The model under review builds one solid part; all positions refer to its coordinate system, in mm. Coordinates: 2 decimals unless noted, no trailing zeros. Loops run counter-clockwise (first coordinate to the right, second up) from the corner with the lowest first, then second, coordinate; pieces in that order, holes last. Notation, with made-up numbers: (64, 36) - (68, 36) arc R26 cw to (68, 67) - close; hole circle Ø9 at (-19.75, 14). An arc over 180 degrees is marked (long way). Answer in a Markdown table with one row per item. Add a question column.
(1) For P1, Ø8, axis at x = 0, y = 118.5, coming from the +Z side; P2, Ø6, axis at x = -118.5, y = 0, coming from the -Z side; P3, Ø1.5, axis at y = -96, z = 4.5, coming from the +X side; P4, Ø1.5, axis at x = -12, z = 1.5, coming from the -Y side, all flat-tipped, find the tip position at first contact; note any pin that passes through.
(2) We need section B-B on x = 25. Write out the cut boundary in (y, z), plus the area to 3 significant figures.
(3) We need section A-A on y = 92.5. Write out the cut boundary in (x, z), plus the area to 3 significant figures.
(4) For line 1 along Y through (x, z) = (0, 2.6); line 2 along Y through (x, z) = (0, 6.25); line 3 along Y through (x, z) = (-32, 6), list the stretches that pass through material, from the lowest coordinate up.
(5) We need section C-C on z = 4.25. Write out the cut boundary in (x, y), plus the area to 3 significant figures.
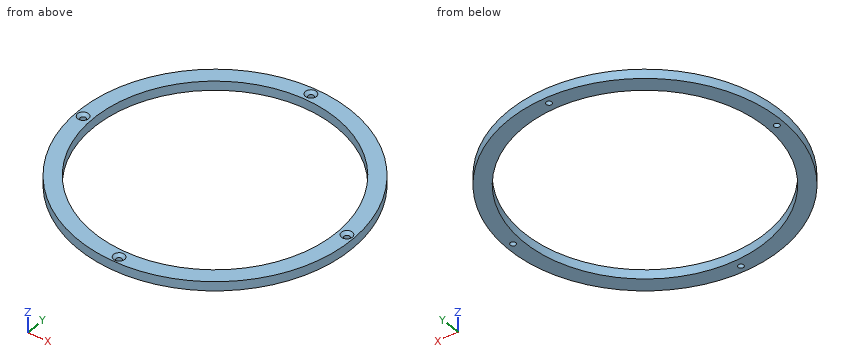
from build123d import *

# Parameters (mm, degrees)
SCHIZZO1_R                                           = 125
SCHIZZO1_R_2                                         = 111
ESTRUSIONE_ESTRUSIONE1_DEPTH                         = 8.5
FORO_SVASATO_PER_VITE_M4_A_TESTA_SVASATA_D           = 5
FORO_SVASATO_PER_VITE_M4_A_TESTA_SVASATA_CSINK_D     = 10
FORO_SVASATO_PER_VITE_M4_A_TESTA_SVASATA_CSINK_ANGLE = 90
RIPETIZIONECIRCOLARE1_COUNT                          = 4


with BuildPart() as part:
    # Schizzo1 → Estrusione-Estrusione1 (new body)
    with BuildSketch(Plane.XY):
        Circle(SCHIZZO1_R)
        Circle(SCHIZZO1_R_2, mode=Mode.SUBTRACT)
    extrude(amount=ESTRUSIONE_ESTRUSIONE1_DEPTH)

    # Foro svasato per Vite M4 a testa svasata cilindrica2 (through all)
    with Locations(Plane.XY.offset(8.5)):
        with Locations((0, -118.5)):
            foro_svasato_per_vite_m4_a_testa_svasata = CounterSinkHole(FORO_SVASATO_PER_VITE_M4_A_TESTA_SVASATA_D / 2, FORO_SVASATO_PER_VITE_M4_A_TESTA_SVASATA_CSINK_D / 2, counter_sink_angle=FORO_SVASATO_PER_VITE_M4_A_TESTA_SVASATA_CSINK_ANGLE)

    # RipetizioneCircolare1: Foro svasato per Vite M4 a testa svasata cilindrica2 ×4 about axis
    ripetizionecircolare1_axis = Axis((0, 0, 0), (0, 0, 1))
    for i in range(1, RIPETIZIONECIRCOLARE1_COUNT):
        add(foro_svasato_per_vite_m4_a_testa_svasata.rotate(ripetizionecircolare1_axis, i * 360 / RIPETIZIONECIRCOLARE1_COUNT), mode=Mode.SUBTRACT)


solid = part.part
Outcome:
| question | item | result |
|---|---|---|
| 1 | P1 | z = 7.5 |
| 1 | P2 | z = 0 |
| 1 | P3 | x = 80.95 |
| 1 | P4 | y = -124.49 |
| 2 | outline | (-122.47, 0) - (-108.15, 0) - (-108.15, 8.5) - (-122.47, 8.5) - close; (108.15, 0) - (122.47, 0) - (122.47, 8.5) - (108.15, 8.5) - close |
| 2 | area | 244 mm² |
| 3 | outline | (-84.08, 0) - (-61.36, 0) - (-61.36, 8.5) - (-84.08, 8.5) - close; (61.36, 0) - (84.08, 0) - (84.08, 8.5) - (61.36, 8.5) - close |
| 3 | area | 386 mm² |
| 4 | line 1 | -125 to -121, -116 to -111, 111 to 116, 121 to 125 |
| 4 | line 2 | -125 to -121.25, -115.75 to -111, 111 to 115.75, 121.25 to 125 |
| 4 | line 3 | -120.83 to -106.29, 106.29 to 120.83 |
| 5 | outline | circle Ø250 at (0, 0); hole circle Ø5 at (-118.5, 0); hole circle Ø222 at (0, 0); hole circle Ø5 at (0, -118.5); hole circle Ø5 at (0, 118.5); hole circle Ø5 at (118.5, 0) |
| 5 | area | 10,300 mm² |
